from build123d import *

# Parameters (mm, degrees)
F0_R     = 1
F1_DEPTH = 2
F3_DEPTH = 2
F5_DEPTH = 60


with BuildPart() as f1:
    # F0 (on Top) → F1 (new body)
    with BuildSketch(Plane.XY):
        with BuildLine():
            Line((-3.7516957595, 3.7800597964), (-3.1099091286, 2.8967162808))
            ThreePointArc((-3.1099091286, 2.8967162808), (-3.4383222261, 2.4980873222), (-3.7159556664, 2.0625647832))
            Line((-3.7159556664, 2.0625647832), (-4.7543882487, 2.3999719824))
            Line((-4.7543882487, 2.3999719824), (-5.8175952323, 2.3207077869))
            Line((-5.8175952323, 2.3207077869), (-6.0706112214, 1.5420046428))
            Line((-6.0706112214, 1.5420046428), (-5.2570490283, 0.8529411765))
            Line((-5.2570490283, 0.8529411765), (-4.218616446, 0.5155339773))
            ThreePointArc((-4.218616446, 0.5155339773), (-4.25, 0), (-4.218616446, -0.5155339773))
            Line((-4.218616446, -0.5155339773), (-5.2570490283, -0.8529411765))
            Line((-5.2570490283, -0.8529411765), (-6.0706112214, -1.5420046428))
            Line((-6.0706112214, -1.5420046428), (-5.8175952323, -2.3207077869))
            Line((-5.8175952323, -2.3207077869), (-4.7543882487, -2.3999719824))
            Line((-4.7543882487, -2.3999719824), (-3.7159556664, -2.0625647832))
            ThreePointArc((-3.7159556664, -2.0625647832), (-3.4383222261, -2.4980873222), (-3.1099091286, -2.8967162808))
            Line((-3.1099091286, -2.8967162808), (-3.7516957595, -3.7800597964))
            Line((-3.7516957595, -3.7800597964), (-4.0048600564, -4.8157237097))
            Line((-4.0048600564, -4.8157237097), (-3.3424555973, -5.29698872))
            Line((-3.3424555973, -5.29698872), (-2.4357127539, -4.7361774161))
            Line((-2.4357127539, -4.7361774161), (-1.793926123, -3.8528339005))
            ThreePointArc((-1.793926123, -3.8528339005), (-1.3133222261, -4.0419901943), (-0.8133222261, -4.1714514209))
            Line((-0.8133222261, -4.1714514209), (-0.8133222261, -5.2633240535))
            Line((-0.8133222261, -5.2633240535), (-0.40938847, -6.25))
            Line((-0.40938847, -6.25), (0.40938847, -6.25))
            Line((0.40938847, -6.25), (0.8133222261, -5.2633240535))
            Line((0.8133222261, -5.2633240535), (0.8133222261, -4.1714514209))
            ThreePointArc((0.8133222261, -4.1714514209), (1.3133222261, -4.0419901943), (1.793926123, -3.8528339005))
            Line((1.793926123, -3.8528339005), (2.4357127539, -4.7361774161))
            Line((2.4357127539, -4.7361774161), (3.3424555973, -5.29698872))
            Line((3.3424555973, -5.29698872), (4.0048600564, -4.8157237097))
            Line((4.0048600564, -4.8157237097), (3.7516957595, -3.7800597964))
            Line((3.7516957595, -3.7800597964), (3.1099091286, -2.8967162808))
            ThreePointArc((3.1099091286, -2.8967162808), (3.4383222261, -2.4980873222), (3.7159556664, -2.0625647832))
            Line((3.7159556664, -2.0625647832), (4.7543882487, -2.3999719824))
            Line((4.7543882487, -2.3999719824), (5.8175952323, -2.3207077869))
            Line((5.8175952323, -2.3207077869), (6.0706112214, -1.5420046428))
            Line((6.0706112214, -1.5420046428), (5.2570490283, -0.8529411765))
            Line((5.2570490283, -0.8529411765), (4.218616446, -0.5155339773))
            ThreePointArc((4.218616446, -0.5155339773), (4.25, 0), (4.218616446, 0.5155339773))
            Line((4.218616446, 0.5155339773), (5.2570490283, 0.8529411765))
            Line((5.2570490283, 0.8529411765), (6.0706112214, 1.5420046428))
            Line((6.0706112214, 1.5420046428), (5.8175952323, 2.3207077869))
            Line((5.8175952323, 2.3207077869), (4.7543882487, 2.3999719824))
            Line((4.7543882487, 2.3999719824), (3.7159556664, 2.0625647832))
            ThreePointArc((3.7159556664, 2.0625647832), (3.4383222261, 2.4980873222), (3.1099091286, 2.8967162808))
            Line((3.1099091286, 2.8967162808), (3.7516957595, 3.7800597964))
            Line((3.7516957595, 3.7800597964), (4.0048600564, 4.8157237097))
            Line((4.0048600564, 4.8157237097), (3.3424555973, 5.29698872))
            Line((3.3424555973, 5.29698872), (2.4357127539, 4.7361774161))
            Line((2.4357127539, 4.7361774161), (1.793926123, 3.8528339005))
            ThreePointArc((1.793926123, 3.8528339005), (1.3133222261, 4.0419901943), (0.8133222261, 4.1714514209))
            Line((0.8133222261, 4.1714514209), (0.8133222261, 5.2633240535))
            Line((0.8133222261, 5.2633240535), (0.40938847, 6.25))
            Line((0.40938847, 6.25), (-0.40938847, 6.25))
            Line((-0.40938847, 6.25), (-0.8133222261, 5.2633240535))
            Line((-0.8133222261, 5.2633240535), (-0.8133222261, 4.1714514209))
            ThreePointArc((-0.8133222261, 4.1714514209), (-1.3133222261, 4.0419901943), (-1.793926123, 3.8528339005))
            Line((-1.793926123, 3.8528339005), (-2.4357127539, 4.7361774161))
            Line((-2.4357127539, 4.7361774161), (-3.3424555973, 5.29698872))
            Line((-3.3424555973, 5.29698872), (-4.0048600564, 4.8157237097))
            Line((-4.0048600564, 4.8157237097), (-3.7516957595, 3.7800597964))
        make_face()
        Circle(F0_R, mode=Mode.SUBTRACT)
    extrude(amount=F1_DEPTH)

    # F2 (on face) → F3 (join)
    with BuildSketch(Plane.XY.offset(2)):
        with BuildLine():
            ThreePointArc((-34.3016055682, -7.25), (-24.9889461736, 4.275), (-15.676286779, -7.25))
            Line((-15.676286779, -7.25), (-14.1722923472, -7.25))
            ThreePointArc((-14.1722923472, -7.25), (-14.1248516042, -3.5262108052), (-15.322638709, 0))
            Line((-15.322638709, 0), (-5.8811097025, 2.1252303477))
            Line((-5.8811097025, 2.1252303477), (-5.8175952323, 2.3207077869))
            Line((-5.8175952323, 2.3207077869), (-4.7543882487, 2.3999719824))
            Line((-4.7543882487, 2.3999719824), (-4.7159827656, 2.3874932845))
            Line((-4.7159827656, 2.3874932845), (-3.2717603315, 2.7125789082))
            ThreePointArc((-3.2717603315, 2.7125789082), (-3.1921627336, 2.8058148696), (-3.1099091286, 2.8967162808))
            Line((-3.1099091286, 2.8967162808), (-3.7516957595, 3.7800597964))
            Line((-3.7516957595, 3.7800597964), (-4.0048600564, 4.8157237097))
            Line((-4.0048600564, 4.8157237097), (-3.3424555973, 5.29698872))
            Line((-3.3424555973, 5.29698872), (-2.4357127539, 4.7361774161))
            Line((-2.4357127539, 4.7361774161), (-1.793926123, 3.8528339005))
            ThreePointArc((-1.793926123, 3.8528339005), (-1.3133222261, 4.0419901943), (-0.8133222261, 4.1714514209))
            Line((-0.8133222261, 4.1714514209), (-0.8133222261, 5.2633240535))
            Line((-0.8133222261, 5.2633240535), (-0.4534381538, 6.1424012594))
            Line((-0.4534381538, 6.1424012594), (-18.8133154383, 3.8528339005))
            ThreePointArc((-18.8133154383, 3.8528339005), (-31.0058393909, 3.958528439), (-35.8056, -7.25))
            Line((-35.8056, -7.25), (-34.3016055682, -7.25))
        make_face()
    extrude(amount=-F3_DEPTH)

    # F4 (on face) → F5 (join)
    with BuildSketch(Plane.XY.offset(2)):
        with BuildLine():
            Line((-15.676286779, -7.25), (-14.1722923472, -7.25))
            ThreePointArc((-14.1722923472, -7.25), (-14.1248516042, -3.5262108052), (-15.322638709, 0))
            ThreePointArc((-15.322638709, 0), (-16.8370854198, 2.1356053409), (-18.8133154383, 3.8528339005))
            ThreePointArc((-18.8133154383, 3.8528339005), (-31.0058393909, 3.958528439), (-35.8056, -7.25))
            Line((-35.8056, -7.25), (-34.3016055682, -7.25))
            ThreePointArc((-34.3016055682, -7.25), (-24.9889461736, 4.275), (-15.676286779, -7.25))
        make_face()
    extrude(amount=F5_DEPTH)


solid = f1.part
Build history of the part. All positions in model axes, mm. A direction names the side the tool comes from. Give positions to 0.01 mm unless a question says otherwise; leave off trailing zeros. Write each loop counter-clockwise with the first axis right and the second up, starting at its lowest first coordinate (ties: lowest second). Pieces come first, ordered by that corner, then holes. Notation, with made-up numbers: (76.25, 85) - (113.25, 85) arc R14 ccw to (113.25, 98) - close; hole circle Ø11 at (-35, 66). An arc over 180 degrees is marked (long way). Use one line per item in the form item = value. Start each with the question number.
1. Band-saw the part on C-C on x = -7. Write the cut outline in (y, z), plus the area to 3 significant figures.
2. Band-saw the part on B-B on x = -27.5. Write the cut outline in (y, z), plus the area to 3 significant figures.
3. Probe line 1 (X direction, y = -5.25, z = 19); line 2 (X direction, y = -3, z = 42.5); line 3 (Y direction, x = 0, z = 1.25). List the from-to ranges inside material, lowest first. Write a range as [from, to].
4. Two-plate mould, pull along X, no slides. Class faces 1 (the face through (-10.668, 1.048, 1.014)), 2 (the face through (-11, 3, 0)): released by +X, released by -X, zero draft, split by the parting line, or undercut.
5. Band-saw the part on A-A on z = 54.5. Write the cut outline in (x, y) (3 decimals), plus the area to 3 significant figures.
6. 3-axis set-ups, long thin cutter, end or side, ignore diameter. For faces 3 (the face through (-9.505, 5.014, 1.014)), 4 (the face through (-15, -7.25, 31)): which of +Z, -Z, +X, -X, +Y, -Y reach the whole face in a straight line?
7. Drop flat-ended pins along their axis: pin 1 Ø0.7 at (x, z) = (0, 1.5) entering from -Y; pin 2 Ø4 at (x, z) = (-26, 14) entering from +Y; pin 3 Ø10 at (x, z) = (-15.5, 23.5) entering from +Y. Give the stop position or say it passes through.
Conclusion:
q1.outline = (1.87, 0) - (5.33, 0) - (5.33, 2) - (1.87, 2) - close
q1.area = 6.91 mm²
q2.outline = (3.94, 0) - (5.46, 0) - (5.46, 62) - (3.94, 62) - close
q2.area = 94.3 mm²
q3.line_1 = [-35.99, -34.51], [-15.46, -13.99]
q3.line_2 = [-35.76, -34.24], [-15.73, -14.22]
q3.line_3 = [-6.25, -1], [1, 6.25]
q4.face_1 = undercut
q4.face_2 = zero draft
q5.outline = (-35.806, -7.25) - (-34.302, -7.25) arc R9.525 cw (long way) to (-15.676, -7.25) - (-14.172, -7.25) arc R11 ccw (long way) to start
q5.area = 53.5 mm²
q6.face_3 = +Z, -Z, +Y
q6.face_4 = +Z, -Z, +X, -X, -Y
q7.pin_1 = -6.25
q7.pin_2 = 5.75
q7.pin_3 = 4.79
